Work out the finished part from the listing and answer in its coordinate system (mm). A direction names the side the tool comes from. Coordinates: 2 decimals unless noted, no trailing zeros. Order: outer loops, then holes, each group sorted by start corner. A loop starts at its lowest first (then second) coordinate and runs counter-clockwise, first axis right, second up. Notation, with made-up numbers: (27, 6) -> (65, 6) arc R25 cw to (65, 25) -> close; hole circle Ø4 at (-15.75, -13.75). An arc over 180 degrees is marked (long way). Answer as CSV lines item,"result". Start each with the question number.
Item 1: For a pull along Y with two mould halves and no side action, classify faces 4 (the face through (4.065, 44.597, -6.108)), 5 (the face through (10, 0.1, -2)), 6 (the face through (10, 27, 0)) as pulls with the +Y half, pulls with the -Y half, needs draft (parallel to the pull), parting line crosses it, or undercut.
Item 2: Each of these flat-tipped pins is pushed along its axis until it touches: pin 1 Ø2.5 at (y, z) = (2, -2) entering from -X; pin 2 Ø11 at (x, y) = (14, 13) entering from -Z; pin 3 Ø4.5 at (x, y) = (9.5, 2.5) entering from -Z. Where does it stop, or does it pass through?
Item 3: Which of the six approach directions +Z, -Z, +X, -X, +Y, -Y give full straight-line access (tool end or side, diameter ignored) to faces 1 (the face through (19.6, 3, -2)), 2 (the face through (14.37, 2.56, -0.76)), 3 (the face through (10, 44.4, -6))?
Item 4: Section B-B (y = 9.5) is taken. Write down the section's boundary in (x, z).
Item 5: Straight lines are drawn through the part: L1, parallel to X at y = 4.25, z = -1.75; L2, parallel to Z at x = 14.5, y = 3.5; L3, parallel to Y at x = 19.75, z = -2. For each, find the intervals that lie inside material, in ascending order.
Item 6: Section A-A (y = 2.5) is taken. Write down the section's boundary in (x, z).
Autodesk Inventor part; units mm, degrees
ref_plane "YZ Plane" through (0, 0, 0) normal (1, 0, 0) x (0, 1, 0)
ref_plane "XZ Plane" through (0, 0, 0) normal (0, 1, 0) x (-1, 0, 0)
ref_plane "XY Plane" through (0, 0, 0) normal (0, 0, 1) x (1, 0, 0)
sketch "Sketch1" plane through (0, 0, 0) normal (0, 0, 1) x (1, 0, 0)
  line L0 (0, 44.4) -> (0, 0) construction
  line L1 (0, 44.4) -> (-0.8, 44.4) construction
  line L2 (-0.8, 44.4) -> (-0.8, -0.8) construction
  line L3 (20.8, -0.8) -> (-0.8, -0.8) construction
  line L4 (20.8, 44.4) -> (20.8, -0.8) construction
  line L5 (20, 44.4) -> (20.8, 44.4) construction
  line L6 (20, 44.4) -> (20, 0) construction
  line L7 (20, 0) -> (0, 0) construction
  line L8 (-0.8, -0.8) -> (20.8, -0.8)
  line L9 (20.8, -0.8) -> (20.8, 44.4)
  line L10 (20.8, 44.4) -> (-0.8, 44.4)
  line L11 (-0.8, 44.4) -> (-0.8, -0.8)
extrude "Extrusion1" add sketch "Sketch1" along normal blind 0.8
sketch "Sketch2" plane through (-0.8, 44.4, 0) normal (0, 1, 0) x (1, 0, 0)
  line L0 (7.1248, 6.15) -> (6.7248, 5.75) construction
  line L1 (7.1248, 10.1) -> (7.1248, 6.15) construction
  line L2 (7.5248, 10.5) -> (7.1248, 10.1) construction
  line L3 (7.5248, 10.5) -> (20.4, 10.5) construction
  line L4 (20.8, 10.1) -> (20.4, 10.5) construction
  line L5 (20.8, 10.1) -> (20.8, 0) construction
  line L6 (20.8, 0) -> (21.6, 0) construction
  line L7 (21.6, 11.1) -> (21.6, 0) construction
  line L8 (21.2, 11.5) -> (21.6, 11.1) construction
  line L9 (21.2, 11.5) -> (0.4, 11.5) construction
  line L10 (0, 11.1) -> (0.4, 11.5) construction
  line L11 (0, 0) -> (0, 11.1) construction
  line L12 (0.8, 0) -> (0, 0) construction
  line L13 (0.8, 0) -> (0.8, 5.35) construction
  line L14 (1.2, 5.75) -> (0.8, 5.35) construction
  line L15 (6.7248, 5.75) -> (1.2, 5.75) construction
  circle A0 centre (4.2195, 7.1194) radius 1 construction
  line L16 (21.6, -0.8) -> (0, -0.8) construction
  line L17 (0, -0.8) -> (21.6, -0.8)
  line L18 (0, -0.8) -> (21.6, -0.8)
  line L19 (21.6, -0.8) -> (21.6, 11.5)
  line L20 (21.6, 11.5) -> (0, 11.5)
  line L21 (0, 11.5) -> (0, -0.8)
  circle A1 centre (4.2195, 7.1194) radius 1.2
  line L22 (14.4, 3.4) -> (14.4, 2.2) construction
  line L23 (13.4, 1.2) -> (14.4, 2.2) construction
  line L24 (13.4, 1.2) -> (8.2, 1.2) construction
  line L25 (7.2, 2.2) -> (8.2, 1.2) construction
  line L26 (7.2, 2.2) -> (7.2, 3.4) construction
  line L27 (7.2, 3.4) -> (14.4, 3.4) construction
  line L28 (7.8, 8.5) -> (7.8, 5.5) construction
  line L29 (7.8, 5.5) -> (0.8, 5.5) construction
  line L30 (0.8, 0) -> (0.8, 5.5) construction
  line L31 (0.8, 0) -> (20.8, 0) construction
  line L32 (20.8, 0) -> (20.8, 8.5) construction
  line L33 (20.8, 8.5) -> (7.8, 8.5) construction
  line L34 (14.6, 3.6) -> (14.6, 2.1172)
  line L35 (14.6, 2.1172) -> (13.4828, 1)
  line L36 (13.4828, 1) -> (8.1172, 1)
  line L37 (8.1172, 1) -> (7, 2.1172)
  line L38 (7, 2.1172) -> (7, 3.6)
  line L39 (7, 3.6) -> (14.6, 3.6)
  dimension "d18" = 0.2
  dimension "d34" = 0.2
extrude "Extrusion2" add sketch "Sketch2" along normal blind 0.8
sketch "Sketch3" plane through (0, 0, 0) normal (0, 0, -1) x (-1, 0, 0)
  line L0 (-20, 0) -> (0, 0) construction
  line L1 (-20, 44.4) -> (-20, 0) construction
  line L2 (0, 44.4) -> (0, 0) construction
  line L3 (-20, 11) -> (-20, 0) construction
  line L4 (0, 11) -> (-20, 11) construction
  line L5 (0, 0) -> (0, 11) construction
  line L6 (-20, 0) -> (0, 0) construction
  line L7 (-19.6, 0.1) -> (-0.4, 0.1)
  line L8 (-0.4, 0.1) -> (-0.4, 4.1)
  line L9 (-0.4, 4.1) -> (-19.6, 4.1)
  line L10 (-19.6, 4.1) -> (-19.6, 0.1)
  dimension "d6" = 4
  dimension "d7" = 0.4
  dimension "d8" = 0.4
  dimension "d9" = 0.1
extrude "Extrusion3" add sketch "Sketch3" along normal blind 3.2
chamfer "Chamfer4" distance 3.2 angle 45 1 edges at (10, 4.1, 0)
sketch "Sketch5" plane through (0.4, 0.1, 0) normal (0, -1, 0) x (1, 0, 0)
  circle A0 centre (14.1, -1.75) radius 1.1
  circle A1 centre (5.1, -1.75) radius 1.1
  circle A2 centre (14.1, -1.75) radius 1
  circle A3 centre (5.1, -1.75) radius 1
  point P0 (-0.4, 0)
  dimension "d33" = 2
extrude "Extrusion5" cut sketch "Sketch5" against normal blind 16.45 contours A2 | A3
chamfer "Chamfer5" distance 0.4 angle 45 11 edges at (-0.8, 22.2, 0.8) (20.8, 22.2, 0.8) (-0.8, 44.8, -11.5) (20.8, 44.8, -11.5) (2.2195, 45.2, -7.1194) (10, 45.2, -3.6) (6.2, 45.2, -2.8586) (6.7586, 45.2, -1.5586) (10, 45.2, -1) (13.2414, 45.2, -1.5586) (13.8, 45.2, -2.8586)
properties part number "carcasainferior"
Checked values:
1,face 4,"needs draft"
1,face 5,"pulls with the -Y half"
1,face 6,"undercut"
2,pin 1,"stops at x = 0.4"
2,pin 2,"stops at z = 0"
2,pin 3,"stops at z = -3.2"
3,face 1,"-Z, +X, -Y"
3,face 2,"-Y"
3,face 3,"-Z, +X, -X"
4,outline,"(-0.8, 0) -> (20.8, 0) -> (20.8, 0.4) -> (20.4, 0.8) -> (-0.4, 0.8) -> (-0.8, 0.4) -> close"
5,L1,"x = 0.4 to 4.5, 6.5 to 13.5, 15.5 to 19.6"
5,L2,"z = -3.2 to -2.75, -0.75 to 0.8"
5,L3,"y = 44.4 to 45.2"
6,outline,"(-0.8, 0) -> (0.4, 0) -> (0.4, -3.2) -> (19.6, -3.2) -> (19.6, 0) -> (20.8, 0) -> (20.8, 0.4) -> (20.4, 0.8) -> (-0.4, 0.8) -> (-0.8, 0.4) -> close; hole circle Ø2 at (5.5, -1.75); hole circle Ø2 at (14.5, -1.75)"
